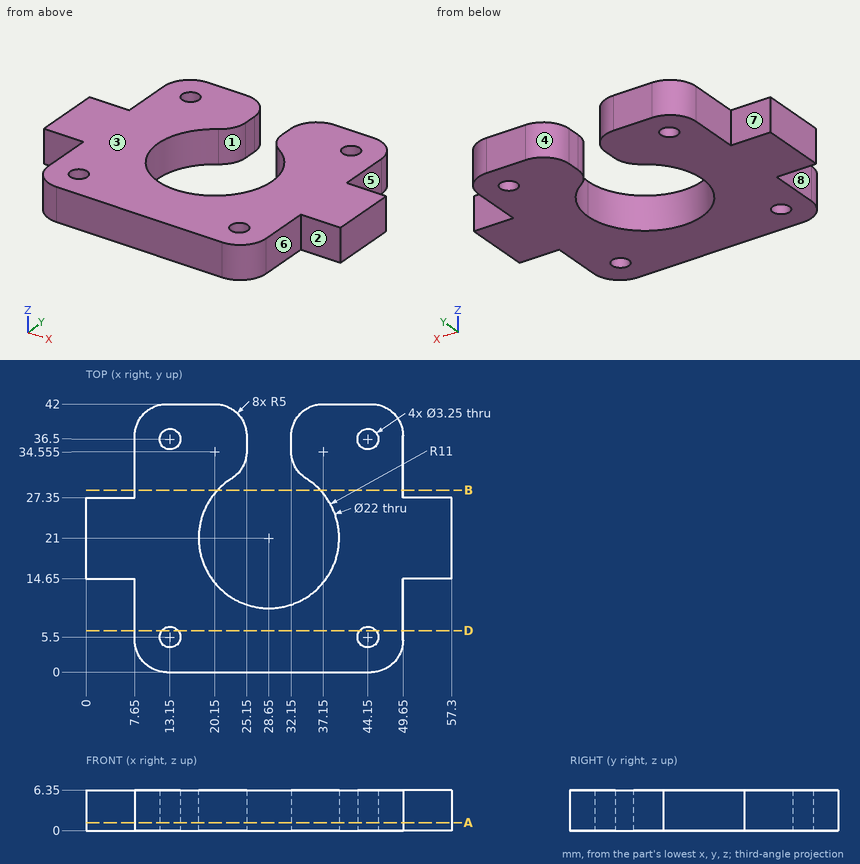
Job drawing, mm, ordinate dimensions from the low corner. One solid piece. A direction names the side the tool comes from. Give positions to 0.01 mm unless a question says otherwise; leave off trailing zeros. Order: outer loops, then holes, each group sorted by start corner. A loop starts at its lowest first (then second) coordinate and runs counter-clockwise, first axis right, second up. Notation, with made-up numbers: M 30,28.5 L 54,28.5 A21 cw 54,61.5 Z; hole C -14,-37 d10. An arc over 180 degrees is marked long. Return JSON: item names as keys, results as strings.
Q1. Two-plate mould, pull along Y, no slides. Class the marked faces 1, 2 and 3: pulls with the +Y half, pulls with the -Y half, needs draft (parallel to the pull), parting line crosses it, or undercut.
Answer list:
{"face 1": "undercut", "face 2": "pulls with the -Y half", "face 3": "needs draft"}
Q2. Wall check: probe 1 along Y at (x, z) = (44.15, 2) (1 decimal); probe 2 along X at (y, z) = (35.5, 3); probe 3 along X at (y, z) = (21, 4.25). Give the ranges that are in metal, low to high. Write a range as from..to.
Answer list:
{"probe 1": "y = 0..3.9, 7.1..34.9, 38.1..42", "probe 2": "x = 7.65..11.87, 14.43..25.15, 32.15..42.87, 45.43..49.65", "probe 3": "x = 0..17.65, 39.65..57.3"}
Q3. 3-axis set-ups, long thin cutter, end or side, ignore diameter. For the marked faces 4, 5, 6, 7 and 8: which of +Z, -Z, +X, -X, +Y, -Y reach the whole face in a straight line?
Answer list:
{"face 4": "+Z, -Z, +Y", "face 5": "+Z, -Z, +X, +Y", "face 6": "+Z, -Z, +X, -Y", "face 7": "+Z, -Z, -X, +Y", "face 8": "+Z, -Z, -X, -Y"}
Q4. Band-saw the part on D-D (y = 6.5). Give the cut face in (x, z).
Answer list:
{"outline": "M 7.65,0 L 11.87,0 L 11.87,6.35 L 7.65,6.35 Z; M 14.43,0 L 42.87,0 L 42.87,6.35 L 14.43,6.35 Z; M 45.43,0 L 49.65,0 L 49.65,6.35 L 45.43,6.35 Z"}
Q5. Band-saw the part on A-A (z = 1.25). Count the separate pieces of the cut face and the enclosed holes in it, then the cut area to 3 significant figures.
Answer list:
{"separate pieces": "1", "enclosed holes": "4", "area": "1,440 mm^2"}
Q6. Band-saw the part on B-B (y = 28.5). Give the cut face in (x, z).
Answer list:
{"outline": "M 7.65,0 L 20.6,0 L 20.6,6.35 L 7.65,6.35 Z; M 36.7,0 L 49.65,0 L 49.65,6.35 L 36.7,6.35 Z"}
Q7. Flat gauge pins, fed straight in: pin 1 (3 mm diameter, centred on x = 28.5, z = 1, fed in from +Y) (1 decimal); pin 2 (2.5 mm diameter, centred on y = 36.5, z = 4, fed in from -X); pin 3 (2.5 mm diameter, centred on y = 36.5, z = 2.5, fed in from +X); pin 4 (17.5 mm diameter, centred on x = 28.65, y = 21, fed in from +Z). Where does each tip first touch, or does it go through?
Answer list:
{"pin 1": "stops at y = 10.1", "pin 2": "stops at x = 7.65", "pin 3": "stops at x = 49.65", "pin 4": "passes through"}
